from build123d import *

# Parameters (mm, degrees)
SKETCH1_W           = 40
SKETCH1_H           = 30
BOSS_EXTRUDE1_DEPTH = 2.85
SKETCH2_R           = 1.5
CUT_EXTRUDE1_DEPTH  = 26.161925602
SKETCH3_R           = 1.5
CUT_EXTRUDE2_DEPTH  = 26.161925602


with BuildPart() as part:
    # Sketch1 → Boss-Extrude1 (new body)
    with BuildSketch(Plane(origin=(0, 0, 0), x_dir=(0, 0, -1), z_dir=(1, 0, 0))):
        Rectangle(SKETCH1_W, SKETCH1_H)
    extrude(amount=BOSS_EXTRUDE1_DEPTH)

    # Sketch2 → Cut-Extrude1 (cut, through all)
    with BuildSketch(Plane(origin=(2.85, 0, 0), x_dir=(0, 0, -1), z_dir=(1, 0, 0))):
        with Locations((-10, 0)):
            Circle(SKETCH2_R)
        with Locations((10, 0)):
            Circle(SKETCH2_R)
    extrude(amount=-CUT_EXTRUDE1_DEPTH, mode=Mode.SUBTRACT)

    # Sketch3 → Cut-Extrude2 (cut, through all)
    with BuildSketch(Plane(origin=(2.85, 0, 0), x_dir=(0, 0, -1), z_dir=(1, 0, 0))):
        with Locations((-15, 11)):
            Circle(SKETCH3_R)
        with Locations((15, 11)):
            Circle(SKETCH3_R)
    cut_extrude2 = extrude(amount=-CUT_EXTRUDE2_DEPTH, mode=Mode.SUBTRACT)

    # Mirror1: Cut-Extrude2 across plane
    add(cut_extrude2.mirror(Plane.ZX), mode=Mode.SUBTRACT)


solid = part.part
Part model, mm, in its own coordinate system. Give positions to 0.01 mm unless a question says otherwise; leave off trailing zeros. Order: outer loops, then holes, each group sorted by start corner. A loop starts at its lowest first (then second) coordinate and runs counter-clockwise, first axis right, second up. Notation, with made-up numbers: (86, -34.75) -> (113, -34.75) arc R25 ccw to (113, -5.75) -> close; hole circle Ø4 at (5, 35.5). An arc over 180 degrees is marked (long way). Use one line per item in the form item = value.
(1) Pull direction Y, two halves, no side cores. Call faces 1 (the face through (1.44, -11.07, -13.5)), 2 (the face through (1, -15, 0)), 3 (the face through (1, 0, 20)), 4 (the face through (1, 15, 0)): +Y half, -Y half, draft (parallel to the pull), parting line (faces both ways), or undercut.
Solution:
face_1 = undercut
face_2 = -Y half
face_3 = draft
face_4 = +Y half
(2) Saw through at C-C (z = -15). Write the cut outline in (x, y), then the cut area to 3 significant figures.
Solution:
outline = (0, -15) -> (2.85, -15) -> (2.85, -12.5) -> (0, -12.5) -> close; (0, -9.5) -> (2.85, -9.5) -> (2.85, 9.5) -> (0, 9.5) -> close; (0, 12.5) -> (2.85, 12.5) -> (2.85, 15) -> (0, 15) -> close
area = 68.4 mm²
(3) Flat gauge pins, fed straight in: P1, Ø2.5, axis at y = -11, z = -15, coming from the +X side; P2, Ø5, axis at y = 0, z = -10, coming from the +X side. Where does each tip first touch, or does it go through?
Solution:
P1 = through
P2 = 2.85
(4) Saw through at A-A (z = 10). Write the cut outline in (x, y).
Solution:
outline = (0, -15) -> (2.85, -15) -> (2.85, -1.5) -> (0, -1.5) -> close; (0, 1.5) -> (2.85, 1.5) -> (2.85, 15) -> (0, 15) -> close
(5) Drill centre lines: line 1 (Y direction, x = 1.55, z = -15); line 2 (Z direction, x = 1.95, y = -11); line 3 (Y direction, x = 1.55, z = -10). Where is each one in solid material? Low to high. Write a range as from..to.
Solution:
line_1 = -15..-12.5, -9.5..9.5, 12.5..15
line_2 = -20..-16.5, -13.5..13.5, 16.5..20
line_3 = -15..-1.5, 1.5..15
(6) Saw through at D-D (x = 1.7). Write the cut outline in (y, z), then the cut area to 3 significant figures.
Solution:
outline = (-15, -20) -> (15, -20) -> (15, 20) -> (-15, 20) -> close; hole circle Ø3 at (-11, -15); hole circle Ø3 at (-11, 15); hole circle Ø3 at (0, -10); hole circle Ø3 at (0, 10); hole circle Ø3 at (11, -15); hole circle Ø3 at (11, 15)
area = 1,160 mm²
(7) Saw through at B-B (y = -11). Write the cut outline in (x, z).
Solution:
outline = (0, -20) -> (2.85, -20) -> (2.85, -16.5) -> (0, -16.5) -> close; (0, -13.5) -> (2.85, -13.5) -> (2.85, 13.5) -> (0, 13.5) -> close; (0, 16.5) -> (2.85, 16.5) -> (2.85, 20) -> (0, 20) -> close
